Geometry check sheet. Reference: the model listing, model coordinates, mm. Coordinates: 2 decimals unless noted, no trailing zeros. Write each loop counter-clockwise with the first axis right and the second up, starting at its lowest first coordinate (ties: lowest second). Pieces come first, ordered by that corner, then holes. Notation, with made-up numbers: (82.25, 49.25) -> (95.25, 49.25) arc R21 ccw to (95.25, 79.25) -> close; hole circle Ø4 at (-33, 36.25). An arc over 180 degrees is marked (long way). One line per question, with ' | ' between items.
```python
from build123d import *

# Parameters (mm, degrees)
SKETCH1_R           = 2.875
SKETCH1_R_2         = 1.5
BOSS_EXTRUDE1_DEPTH = 3
CUT_EXTRUDE1_DEPTH  = 10
SKETCH3_R           = 1.42
CUT_EXTRUDE2_DEPTH  = 20
FILLET3_R           = 10
FILLET5_R           = 10
FILLET6_R           = 10


with BuildPart() as part:
    # Sketch1 → Boss-Extrude1 (new body)
    with BuildSketch(Plane(origin=(0, 0, 0), x_dir=(1, 0, 0), z_dir=(0, 1, 0))):
        with BuildLine():
            Line((-61.421696796, 42.03125), (-67.039661146, 35))
            Line((-67.039661146, 35), (-74.713671979, 35))
            Line((-74.713671979, 35), (-98.423870832, 17.924994351))
            ThreePointArc((-98.423870832, 17.924994351), (-101.259728964, -30.910949772), (-54.215728753, -17.5))
            Line((-54.215728753, -17.5), (37.189110868, -17.5))
            ThreePointArc((37.189110868, -17.5), (97.810889132, -17.5), (67.5, 35))
            Line((67.5, 35), (61.88203565, 42.03125))
            Line((61.88203565, 42.03125), (-61.421696796, 42.03125))
        make_face()
        with Locations(Location((-97.810889132, -17.5, 0), (0, 0, 270))):
            Circle(SKETCH1_R, mode=Mode.SUBTRACT)
        with Locations(Location((52.189110868, -17.5, 0), (0, 0, 270))):
            Circle(SKETCH1_R_2, mode=Mode.SUBTRACT)
    extrude(amount=BOSS_EXTRUDE1_DEPTH)

    # Sketch2 → Cut-Extrude1 (cut)
    with BuildSketch(Plane(origin=(0, 3, 0), x_dir=(1, 0, 0), z_dir=(0, 1, 0))):
        with BuildLine():
            Line((-47.810889132, 16.294274109), (27.189110868, 16.294274109))
            ThreePointArc((27.189110868, 16.294274109), (36.042740422, 7.440644555), (27.189110868, -1.412984999))
            Line((27.189110868, -1.412984999), (-47.810889132, -1.412984999))
            ThreePointArc((-47.810889132, -1.412984999), (-56.664518687, 7.440644555), (-47.810889132, 16.294274109))
        make_face()
    extrude(amount=-CUT_EXTRUDE1_DEPTH, mode=Mode.SUBTRACT)

    # Sketch3 → Cut-Extrude2 (cut)
    with BuildSketch(Plane(origin=(0, 3, 0), x_dir=(1, 0, 0), z_dir=(0, 1, 0))):
        with Locations(Location((-28.142811364, -10.5, 0), (0, 0, 270))):
            Circle(SKETCH3_R)
        with Locations(Location((23.088594579, -10.5, 0), (0, 0, 270))):
            Circle(SKETCH3_R)
        with Locations(Location((-28.142811364, 38.03125, 0), (0, 0, 270))):
            Circle(SKETCH3_R)
        with Locations(Location((23.088594579, 38.03125, 0), (0, 0, 270))):
            Circle(SKETCH3_R)
    extrude(amount=-CUT_EXTRUDE2_DEPTH, mode=Mode.SUBTRACT)

    # Sketch6 → Loft1 section 0
    with BuildSketch(Plane(origin=(0, 3, 0), x_dir=(1, 0, 0), z_dir=(0, 1, 0)), mode=Mode.PRIVATE) as loft1_s0:
        with BuildLine():
            Line((72, 15.450849719), (75.63271264, 5))
            Line((75.63271264, 5), (86.694631307, 4.774575141))
            Line((86.694631307, 4.774575141), (77.877852523, -1.909830056))
            Line((77.877852523, -1.909830056), (81.0817816, -12.5))
            Line((81.0817816, -12.5), (72, -6.180339887))
            Line((72, -6.180339887), (62.9182184, -12.5))
            Line((62.9182184, -12.5), (66.122147477, -1.909830056))
            Line((66.122147477, -1.909830056), (57.305368693, 4.774575141))
            Line((57.305368693, 4.774575141), (68.36728736, 5))
            Line((68.36728736, 5), (72, 15.450849719))
        make_face()
    loft([Vertex(72, 6, 0), loft1_s0.sketch])

    # Fillet3
    fillet3_edges = [part.edges().sort_by_distance(p)[0] for p in [
        (37.189110868, 1.5, 17.5),
        (-54.215728753, 1.5, 17.5),
    ]]
    fillet(fillet3_edges, radius=FILLET3_R)

    # Fillet5
    fillet5_edges = [part.edges().sort_by_distance(p)[0] for p in [
        (-67.039661146, 1.5, -35),
        (67.5, 1.5, -35),
    ]]
    fillet(fillet5_edges, radius=FILLET5_R)

    # Fillet6
    fillet6_edges = [part.edges().sort_by_distance(p)[0] for p in [
        (61.88203565, 1.5, -42.03125),
        (-61.421696796, 1.5, -42.03125),
        (-74.713671979, 1.5, -35),
    ]]
    fillet(fillet6_edges, radius=FILLET6_R)


solid = part.part
```
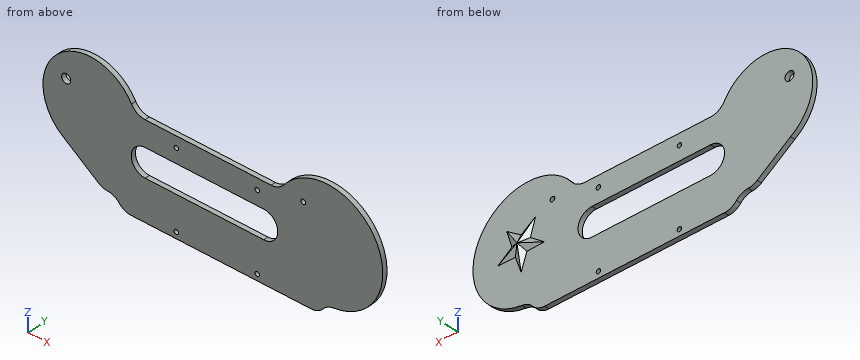
(1) Cross-section at D-D (x = -82.5). Record the cut outline in (y, z).
Answers below:
outline: (0, -29.39) -> (3, -29.39) -> (3, 37.5) -> (0, 37.5) -> close
(2) Material ranges on line 1 (X direction, y = 1.1, z = 10.5); line 2 (Z direction, x = 16, y = 0.75); line 3 (Y direction, x = 87, z = 24), recorded low to high.
Answers below:
line 1: x = -112.35 to -29.56, -26.72 to 21.67, 24.51 to 100.89 | line 2: z = -42.03 to -16.29, 1.41 to 17.5 | line 3: y = 0 to 3
(3) Cross-section at A-A (x = -18). Record the cut outline in (y, z).
Answers below:
outline: (0, -42.03) -> (3, -42.03) -> (3, -16.29) -> (0, -16.29) -> close; (0, 1.41) -> (3, 1.41) -> (3, 17.5) -> (0, 17.5) -> close
(4) Cross-section at C-C (y = 1.25). Count the separate pieces of the cut face and the enclosed holes in it, plus the area to 3 significant figures.
Answers below:
separate pieces: 1 | enclosed holes: 7 | area: 11,300 mm²
(5) Cross-section at B-B (z = -2). Record the cut outline in (x, y).
Answers below:
outline: (-110.96, 0) -> (-54.8, 0) -> (-54.8, 3) -> (-110.96, 3) -> close; (34.17, 0) -> (102.44, 0) -> (102.44, 3) -> (83.03, 3) -> (78.16, 4.74) -> (73.45, 4.8) -> (72, 5.61) -> (70.55, 4.8) -> (65.84, 4.74) -> (60.97, 3) -> (34.17, 3) -> close
(6) Depth check by flat-ended pin: P1, Ø24, axis at x = 1.5, z = -17, coming from the +Y side; P2, Ø0.9, axis at x = -25.5, y = 2, coming from the +Z side; P3, Ø1.5, axis at y = 2, z = 20, coming from the -X side. Enter the tip coordinate at first touch or a pass-through.
Answers below:
P1: stops at y = 3 | P2: stops at z = 17.5 | P3: stops at x = -110.1
